Here's how the part is built. I have some questions about the finished solid (model axes, mm). A direction names the side the tool comes from. Round coordinates to 2 decimals unless told otherwise and drop trailing zeros. Write each loop counter-clockwise with the first axis right and the second up, starting at its lowest first coordinate (ties: lowest second). Pieces come first, ordered by that corner, then holes. Notation, with made-up numbers: (-34, 56) -> (0, 56) arc R33 ccw to (0, 95) -> close; hole circle Ø8 at (66.5, -13). An arc over 180 degrees is marked (long way). Answer as CSV lines item,"result".
Autodesk Inventor part; units mm, degrees
ref_plane "工作平面1" through (40, 100, 45.1945) normal (0.5, -0.866, 0) x (0, 0, -1)
ref_plane "工作平面2" through (-50, 100, -47.95) normal (-0.4226, -0.9063, 0) x (0, 0, 1)
ref_plane "YZ Plane" through (0, 0, 0) normal (1, 0, 0) x (0, 1, 0)
sketch "草图1" plane through (0, 0, 0) normal (0, 1, 0) x (-1, 0, 0)
  circle A0 centre (0, 0) radius 13.45
  dimension "d0" = 26.9
extrude "拉伸1" add sketch "草图1" along normal blind 100
sketch "草图2" plane through (0, 100, 0) normal (0, 1, 0) x (1, 0, 0)
  line L0 (40, -45.1945) -> (40, 45.1945)
  line L1 (0, 0) -> (40, 0) construction
  line L2 (-50, 47.95) -> (-50, -45.1945)
  dimension "d3" = 40
  dimension "d7" = 50
ref_plane "工作平面1" through (40, 100, 45.1945) normal (0.5, -0.866, 0) x (0, 0, -1)
sketch "草图3" plane through (40, 100, 45.1945) normal (0.5, -0.866, 0) x (0, 0, -1)
  circle A0 centre (45.1945, -47.9023) radius 13.45
  line L0 (31.7445, -84.641) -> (31.7445, -34.641)
  line L1 (58.6445, -84.641) -> (58.6445, -34.641)
  point P0 (45.1945, -84.641)
extrude "拉伸2" add sketch "草图3" against normal blind 60
ref_plane "工作平面2" through (-50, 100, -47.95) normal (-0.4226, -0.9063, 0) x (0, 0, 1)
sketch "草图4" plane through (-50, 100, -47.95) normal (-0.4226, -0.9063, 0) x (0, 0, 1)
  circle A0 centre (47.95, -56.336) radius 13.45
  line L0 (61.4, -87.5772) -> (61.4, -45.3154)
  line L1 (34.5, -87.5772) -> (34.5, -45.3154)
  point P0 (47.95, -87.5772)
extrude "拉伸3" add sketch "草图4" against normal blind 70
properties part number "珊瑚" material "聚苯乙烯"
1. On a 3-axis mill with a long thin cutter (end or side, diameter ignored), from which of +Z, -Z, +X, -X, +Y, -Y can I reach the whole of each face in a straight line? I mean faces 4 (the face through (-1, 100, -10)), 5 (the face through (-1, 100, 11)), 6 (the face through (-27.646, 95.101, 2.916)). Say none if no direction works.
Numbers:
face 4,"-Z, +Y"
face 5,"+Z, +Y"
face 6,"none"
2. If we mould it in two halves opening along X, with no side actions, what happens to faces 1 (the face through (-5.914, 73.491, -12.249)), 2 (the face through (0, 0, 0)), 3 (the face through (30.5, 139.7, -0.2))? For each: released by +X, released by -X, zero draft, split by the parting line, or undercut.
Numbers:
face 1,"undercut"
face 2,"zero draft"
face 3,"released by +X"
3. Suppose I cut it at B-B on z = -2.5. Please give me the cut outline in (x, y), and give its area (3 significant figures).
Numbers:
outline,"(-42.93, 121.4) -> (-13.22, 69.94) -> (-13.22, 0) -> (13.22, 0) -> (13.22, 70.99) -> (42.62, 134.05) -> (18.66, 145.22) -> (-1.36, 102.27) -> (-20.04, 134.62) -> close"
area,"5,110 mm^2"
4. Suppose I cut it at A-A on y = 60. Please give me the cut outline in (x, z), and give its area (3 significant figures).
Numbers:
outline,"circle Ø26.9 at (0, 0)"
area,"568 mm^2"
5. For pin 1 Ø2 at (x, z) = (26, -3.5) entering from -Y; pin 2 Ø10 at (y, z) = (17.5, 5) entering from +X; pin 3 Ø8 at (y, z) = (111.5, 8) entering from +X, each with a flat end and sliding along its axis, tell me the tip position at first contact or that it passes through.
Numbers:
pin 1,"stops at y = 96.72"
pin 2,"stops at x = 13.45"
pin 3,"stops at x = 32.54"
6. If I drill on line 1 (X direction, y = 104, z = -8); line 2 (Y direction, x = -1, z = 11.25); line 3 (X direction, y = 113, z = 1.25), over which ranges is the centre line in solid material (lowest first)?
Numbers:
line 1,"x = -30.11 to -5.14, 2.1 to 25.96"
line 2,"y = 0 to 100"
line 3,"x = -38.28 to -7.35, 3.45 to 33"
